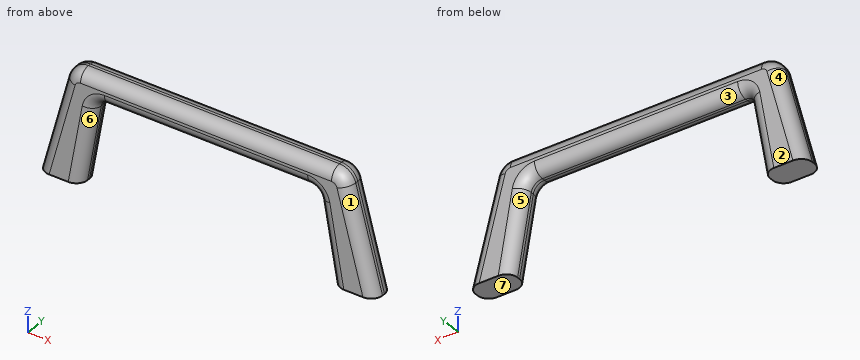
from build123d import *

# Parameters (mm, degrees)
F1_DEPTH = 22.5
F2_R     = 30
F3_R     = 20
F4_R     = 20


with BuildPart() as f1:
    # F0 (on Front) → F1 (new body, symmetric)
    with BuildSketch(Plane.XZ):
        Polygon((-246.410162, 200), (-300, 0), (-225, 0), (-197.669318, 155), (197.669318, 155), (225, 0), (300, 0), (246.410162, 200), align=None)
    extrude(amount=F1_DEPTH, both=True)

    # F2
    f2_edges = [f1.edges().sort_by_distance(p)[0] for p in [
        (246.410162, 0, 200),
        (-246.410162, 0, 200),
    ]]
    fillet(f2_edges, radius=F2_R)

    # F3
    f3_edges = [f1.edges().sort_by_distance(p)[0] for p in [
        (-197.669318, 0, 155),
        (197.669318, 0, 155),
    ]]
    fillet(f3_edges, radius=F3_R)

    # F4
    f4_edges = [f1.edges().sort_by_distance(p)[0] for p in [
        (0, 22.5, 200),
        (0, 22.5, 155),
        (212.79174, -22.5, 69.236482),
        (276.184063, -22.5, 88.882286),
    ]]
    fillet(f4_edges, radius=F4_R)


solid = f1.part
Verification items for the finished model (mm, model axes). Face numbers are marked on the shaded views. A direction names the side the tool comes from. Coordinates: 2 decimals unless noted, no trailing zeros. Order: outer loops, then holes, each group sorted by start corner. A loop starts at its lowest first (then second) coordinate and runs counter-clockwise, first axis right, second up.
Item 1: Depth check by flat-ended pin: pin 1 (4 mm diameter, centred on y = 3.5, z = 175, fed in from -X); pin 2 (8 mm diameter, centred on y = -16.5, z = 85.5, fed in from -X); pin 3 (8 mm diameter, centred on y = 14.5, z = 70.5, fed in from +X). Enter the tip coordinate at first touch or a pass-through.
Filled in:
pin 1: stops at x = -253.63
pin 2: stops at x = -274.54
pin 3: stops at x = 279.67
Item 2: Access from +Z, -Z, +X, -X, +Y, -Y to the whole of each face (thin tool, end or side, straight path). Record for the marked faces 5, 6 and 7.
Filled in:
face 5: -Z, +Y
face 6: -Z, -Y
face 7: -Z, +X, -X, +Y, -Y
Item 3: Section check A-A, the plane x = 151.5. Enter the section's corners in (y, z).
Filled in:
outline: (-22.5, 175) arc R20 ccw to (-2.5, 155) - (2.5, 155) arc R20 ccw to (22.5, 175) - (22.5, 180) arc R20 ccw to (2.5, 200) - (-2.5, 200) arc R20 ccw to (-22.5, 180) - close
Item 4: Release check for a two-part mould opening along X. For the marked faces 1, 2, 3 and 4 record: +X half, -X half, draft (parallel to the pull), parting line (faces both ways), or undercut.
Filled in:
face 1: +X half
face 2: draft
face 3: undercut
face 4: -X half
Item 5: Material ranges on L1, parallel to X at y = 8.5, z = 102; L2, parallel to X at y = -7.5, z = 81; L3, parallel to Z at x = -32.5, y = -2, recorded low to high.
Filled in:
L1: x = -271.72 to -207.95, 207.95 to 271.72
L2: x = -277.64 to -211.36, 211.36 to 277.64
L3: z = 155 to 200
